Could you check a few things on this model? Use its own coordinates, in mm. A direction names the side the tool comes from. Coordinates: 2 decimals unless noted, no trailing zeros. Order: outer loops, then holes, each group sorted by start corner. A loop starts at its lowest first (then second) coordinate and runs counter-clockwise, first axis right, second up. Notation, with made-up numbers: M 54.5,84.25 L 96.5,84.25 A25 ccw 96.5,116.25 Z; hole C 80.5,48.5 d7. An arc over 180 degrees is marked long. Write item = value, one per line. Start each with the question number.
from build123d import *

# Parameters (mm, degrees)
SKETCH1_R           = 14.2875
BOSS_EXTRUDE1_DEPTH = 7.9248
SKETCH2_R           = 15.8623
SKETCH2_R_2         = 14.2875
BOSS_EXTRUDE2_DEPTH = 1.5748


with BuildPart() as part:
    # Sketch1 → Boss-Extrude1 (new body)
    with BuildSketch(Plane(origin=(0, 0, 0), x_dir=(1, 0, 0), z_dir=(0, 1, 0))):
        Circle(SKETCH1_R)
        Polygon((-3.666174209, 6.35), (-7.332348419, 0), (-3.666174209, -6.35), (3.666174209, -6.35), (7.332348419, 0), (3.666174209, 6.35), align=None, mode=Mode.SUBTRACT)
    extrude(amount=BOSS_EXTRUDE1_DEPTH)

    # Sketch2 → Boss-Extrude2 (add)
    with BuildSketch(Plane(origin=(0, 7.9248, 0), x_dir=(1, 0, 0), z_dir=(0, 1, 0))):
        Circle(SKETCH2_R)
        Circle(SKETCH2_R_2, mode=Mode.SUBTRACT)
    extrude(amount=-BOSS_EXTRUDE2_DEPTH)


solid = part.part
(1) Imagine slicing it at D-D on x = 13. List the corners of the cut face in (y, z) for me, plus the area to 3 significant figures.
(2) Thinking about a two-plate mould opening in X: for faces 4 (the flat face through (5.474, 3.907, 3.219)), 5 (the flat face through (0, 7.925, 7)), 6 (the cylindrical face through (-14.274, 3.131, -0.628)), which applies, released by +X, released by -X, zero draft, split by the parting line, or undercut?
(3) For faces 1 (the flat face through (0, 0, -7)), 2 (the flat face through (-11.82, 6.35, -8.3)), 3 (the flat face through (-5.474, 3.907, -3.219)), which set-ups out of +Z, -Z, +X, -X, +Y, -Y let a thin tool reach every point of the face, with its end or its side?
(4) Please list where these lines run through material, in increasing order: probe 1 along X at (y, z) = (1.5, 0); probe 2 along Y at (x, z) = (-13, -6); probe 3 along X at (y, z) = (2, -5.5). Write a range as from..to.
(5) Imagine slicing it at C-C on z = 1.5. List the corners of the cut face in (x, y) for me.
(6) Imagine slicing it at B-B on x = 0. List the corners of the cut face in (y, z) for me.
(7) Will these pins go through, and if not, where does the flat tip stop? P1, Ø3, axis at x = -4.5, z = 1.5, coming from the +Y side; P2, Ø3, axis at y = 7, z = 5.5, coming from the +X side; P3, Ø1, axis at y = 2.5, z = -3.5, coming from the +X side; P4, Ø1, axis at x = 6.5, z = -8, coming from the -Y side.
Response:
q1.outline = M 0,-5.93 L 6.35,-5.93 L 6.35,-9.09 L 7.92,-9.09 L 7.92,9.09 L 6.35,9.09 L 6.35,5.93 L 0,5.93 Z
q1.area = 104 mm2
q2.face_4 = undercut
q2.face_5 = zero draft
q2.face_6 = split by the parting line
q3.face_1 = +Z, -Z, +X, -X, -Y
q3.face_2 = -Y
q3.face_3 = +Y, -Y
q4.probe_1 = -14.29..-7.33, 7.33..14.29
q4.probe_2 = 6.35..7.92
q4.probe_3 = -13.19..-4.16, 4.16..13.19
q5.outline = M -15.79,6.35 L -14.21,6.35 L -14.21,0 L -6.47,0 L -6.47,7.92 L -15.79,7.92 Z; M 6.47,0 L 14.21,0 L 14.21,6.35 L 15.79,6.35 L 15.79,7.92 L 6.47,7.92 Z
q6.outline = M 0,-14.29 L 6.35,-14.29 L 6.35,-15.86 L 7.92,-15.86 L 7.92,-6.35 L 0,-6.35 Z; M 0,6.35 L 7.92,6.35 L 7.92,15.86 L 6.35,15.86 L 6.35,14.29 L 0,14.29 Z
q7.P1 = through
q7.P2 = 15.35
q7.P3 = 13.97
q7.P4 = 0
